from build123d import *

# Parameters (mm, degrees)
ESBO_O1_R                = 39.5
ESBO_O1_R_2              = 3.5
RESSALTO_EXTRUS_O1_DEPTH = 5
CHANFRO1_SIZE            = 1


with BuildPart() as part:
    # Esboço1 → Ressalto-extrusão1 (new body)
    with BuildSketch(Plane(origin=(0, 0, 0), x_dir=(1, 0, 0), z_dir=(0, 1, 0))):
        with Locations(Location((0, 0, 0), (0, 0, 270))):
            Circle(ESBO_O1_R)
        with Locations(Location((-21.213203436, 21.213203436, 0), (0, 0, 270))):
            Circle(ESBO_O1_R_2, mode=Mode.SUBTRACT)
        with Locations(Location((-21.213203436, -21.213203436, 0), (0, 0, 270))):
            Circle(ESBO_O1_R_2, mode=Mode.SUBTRACT)
        with Locations(Location((21.213203436, -21.213203436, 0), (0, 0, 270))):
            Circle(ESBO_O1_R_2, mode=Mode.SUBTRACT)
        with Locations(Location((21.213203436, 21.213203436, 0), (0, 0, 270))):
            Circle(ESBO_O1_R_2, mode=Mode.SUBTRACT)
        with Locations(Location((-30, 0, 0), (0, 0, 270))):
            Circle(ESBO_O1_R_2, mode=Mode.SUBTRACT)
        with Locations(Location((0, -30, 0), (0, 0, 270))):
            Circle(ESBO_O1_R_2, mode=Mode.SUBTRACT)
        with Locations(Location((30, 0, 0), (0, 0, 270))):
            Circle(ESBO_O1_R_2, mode=Mode.SUBTRACT)
        with Locations(Location((0, 30, 0), (0, 0, 270))):
            Circle(ESBO_O1_R_2, mode=Mode.SUBTRACT)
    extrude(amount=RESSALTO_EXTRUS_O1_DEPTH)

    # Chanfro1
    chanfro1_edges = [part.edges().sort_by_distance(p)[0] for p in [
        (0, 0, -33.5),
        (30, 0, -3.5),
        (-21.213203436, 5, -24.713203436),
        (0, 0, 26.5),
        (-30, 0, -3.5),
        (21.213203436, 0, -24.713203436),
        (21.213203436, 0, 17.713203436),
        (-21.213203436, 0, 17.713203436),
        (-21.213203436, 0, -24.713203436),
        (-21.213203436, 5, 17.713203436),
        (21.213203436, 5, 17.713203436),
        (21.213203436, 5, -24.713203436),
        (-30, 5, -3.5),
        (0, 5, 26.5),
        (30, 5, -3.5),
        (0, 5, -33.5),
    ]]
    chamfer(chanfro1_edges, length=CHANFRO1_SIZE)


solid = part.part
Geometry check sheet. Reference: the model listing, model coordinates, mm. Round coordinates to 2 decimals unless told otherwise and drop trailing zeros. Write each loop counter-clockwise with the first axis right and the second up, starting at its lowest first coordinate (ties: lowest second). Pieces come first, ordered by that corner, then holes.
Item 1: Go/stop test with flat-tipped pins: pin 1 Ø3 at (x, y) = (-11.5, 1.5) entering from -Z; pin 2 Ø5.5 at (x, z) = (21.21, -21.21) entering from +Y; pin 3 Ø1.5 at (x, y) = (-21.5, 3) entering from -Z; pin 4 Ø8 at (x, z) = (0, 30) entering from -Y. Record where each tip stops, or that it passes through.
Determined:
pin 1: stops at z = -38.21
pin 2: passes through
pin 3: stops at z = -33.61
pin 4: stops at y = 0.5
Item 2: Section check D-D (y = 2.1). Give the number of separate pieces and of enclosed holes in the cut face, plus the area to 3 significant figures.
Determined:
separate pieces: 1
enclosed holes: 8
area: 4,590 mm2
Item 3: Mould release check, pull along Z, two halves, no side actions. Record for faces 1 (the face through (11.865, 2.465, 37.676)), 2 (the face through (22.265, 2.479, -17.875)), 3 (the face through (1, 5, -1)): +Z half, -Z half, draft (parallel to the pull), parting line (faces both ways), or undercut.
Determined:
face 1: parting line
face 2: undercut
face 3: draft
Item 4: Section check B-B (z = 0). Record the boundary of the cut face in (x, y), plus the area to 3 significant figures.
Determined:
outline: (-39.5, 0) - (-34.5, 0) - (-33.5, 1) - (-33.5, 4) - (-34.5, 5) - (-39.5, 5) - close; (-26.5, 1) - (-25.5, 0) - (25.5, 0) - (26.5, 1) - (26.5, 4) - (25.5, 5) - (-25.5, 5) - (-26.5, 4) - close; (33.5, 1) - (34.5, 0) - (39.5, 0) - (39.5, 5) - (34.5, 5) - (33.5, 4) - close
area: 321 mm2
Item 5: Section check C-C (x = 30). Record the boundary of the cut face in (y, z).
Determined:
outline: (0, -25.7) - (5, -25.7) - (5, -4.5) - (4, -3.5) - (1, -3.5) - (0, -4.5) - close; (0, 4.5) - (1, 3.5) - (4, 3.5) - (5, 4.5) - (5, 25.7) - (0, 25.7) - close
Item 6: Material ranges on line 1 along X through (y, z) = (3.4, -22); line 2 along Z through (x, y) = (-2, 2.65); line 3 along X through (y, z) = (0.25, 20.5), recorded low to high.
Determined:
line 1: x = -32.81 to -24.62, -17.8 to 17.8, 24.62 to 32.81
line 2: z = -39.45 to -32.87, -27.13 to 27.13, 32.87 to 39.45
line 3: x = -33.76 to -25.4, -17.02 to 17.02, 25.4 to 33.76
Item 7: Section check A-A (x = 0). Record the boundary of the cut face in (y, z), plus the area to 3 significant figures.
Determined:
outline: (0, -39.5) - (5, -39.5) - (5, -34.5) - (4, -33.5) - (1, -33.5) - (0, -34.5) - close; (0, -25.5) - (1, -26.5) - (4, -26.5) - (5, -25.5) - (5, 25.5) - (4, 26.5) - (1, 26.5) - (0, 25.5) - close; (0, 34.5) - (1, 33.5) - (4, 33.5) - (5, 34.5) - (5, 39.5) - (0, 39.5) - close
area: 321 mm2
